Could you check a few things on this drawing? It's one solid part, dimensions in mm from its lowest x, y, z. A direction names the side the tool comes from. Coordinates: 2 decimals unless noted, no trailing zeros.
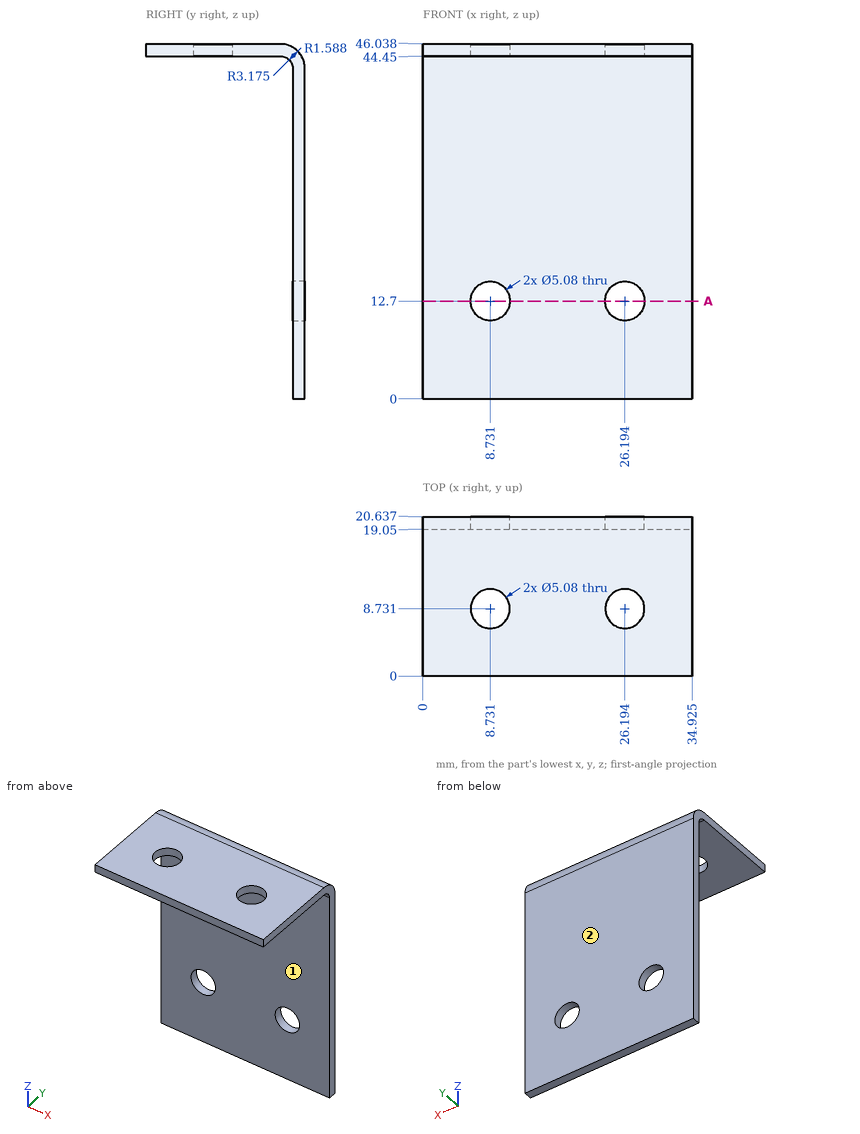
Q1. For the marked faces 1 and 2, which set-ups out of +Z, -Z, +X, -X, +Y, -Y let a thin tool reach every point of the face, with its end or its side?
Q2. If we section it at A-A on z = 12.7: Give the number of separate pieces and of enclosed holes in the cut face.
Q3. I need wall thicknesses on L1, parallel to X at y = 20, z = 12.7 (1 decimal); L2, parallel to Z at x = 31.5, y = 6.5; L3, parallel to Y at x = 30, z = 30. Which ranges of each line are inside material? Lowest first, please.
Q4. Will these pins go through, and if not, where does the flat tip stop? pin 1 (3 mm diameter, centred on x = 8.73, y = 8.73, fed in from -Z); pin 2 (5 mm diameter, centred on x = 31, z = 31.5, fed in from -Y); pin 3 (1 mm diameter, centred on x = 21.5, y = 7.5, fed in from -Z).
Reply:
1. face 1: -Z, +X, -X, -Y
1. face 2: +Z, -Z, +X, -X, +Y
2. separate pieces: 3
2. enclosed holes: 0
3. L1: x = 0 to 6.2, 11.3 to 23.7, 28.7 to 34.9
3. L2: z = 44.45 to 46.04
3. L3: y = 19.05 to 20.64
4. pin 1: passes through
4. pin 2: stops at y = 19.05
4. pin 3: stops at z = 44.45
